Geometry check sheet. Reference: the model listing, model coordinates, mm. Face numbers are marked on the shaded views. A direction names the side the tool comes from. Give positions to 0.01 mm unless a question says otherwise; leave off trailing zeros. Write each loop counter-clockwise with the first axis right and the second up, starting at its lowest first coordinate (ties: lowest second). Pieces come first, ordered by that corner, then holes. Notation, with made-up numbers: M -6.75,27 L -0.75,27 A15 cw -0.75,52 Z; hole C 12.5,5 d9. An arc over 180 degrees is marked long. One line per item, written item: value. Start each with the question number.
1. Cross-section at A-A on z = -3. Record the cut outline in (x, y), then the cut area to 3 significant figures.
2. Tool access check on the marked faces 4 and 5. Record the directions out of +Z, -Z, +X, -X, +Y, -Y that give a thin tool (end or side, any length) a straight path to the whole face; none if there is none.
3. Scan lines: line 1 (Z direction, x = -2, y = -6.75); line 2 (Z direction, x = -2.5, y = -3.75); line 3 (Y direction, x = -0.25, z = -9). Record each from-to range of solid material in increasing order.
4. Release check for a two-part mould opening along Z. For the marked faces 1, 2 and 3 record: pulls with the +Z half, pulls with the -Z half, needs draft (parallel to the pull), parting line crosses it, or undercut.
5. Gauge pin test, flat ends, axial feed: pin 1 (3 mm diameter, centred on y = -1.5, z = -5, fed in from +X); pin 2 (6 mm diameter, centred on x = -4.5, y = 2, fed in from +Z); pin 3 (1 mm diameter, centred on y = 0, z = -4.5, fed in from -X). Record the tip position at first contact, or that the pin passes through.
from build123d import *

# Parameters (mm, degrees)
SKETCH_2_R          = 1.5
CUT_EXTRUDE_1_DEPTH = 24.941073563


with BuildPart() as part:
    # Эскиз1 → Повернуть1 (revolve)
    with BuildSketch(Plane(origin=(0, 0, 0), x_dir=(0, 0, -1), z_dir=(1, 0, 0)), mode=Mode.PRIVATE) as revolve_1_sk:
        with BuildLine():
            Line((-16.75, 0), (16.75, 0))
            Line((16.75, 0), (16.75, 5.5))
            Line((16.75, 5.5), (11.95, 5.5))
            Line((11.95, 5.5), (10.75, 7.65))
            Line((10.75, 7.65), (8.75, 7.65))
            Line((8.75, 7.65), (8.75, 4))
            Line((8.75, 4), (2.45, 4))
            Line((2.45, 4), (2.45, 7.65))
            Line((2.45, 7.65), (1.45, 7.65))
            Line((1.45, 7.65), (1.45, 6.5))
            ThreePointArc((1.45, 6.5), (-6.880526727, 5.027063991), (-14.723327208, 1.855676812))
            ThreePointArc((-14.723327208, 1.855676812), (-15.854421467, 1.056447361), (-16.75, 0))
        make_face()
    revolve(revolve_1_sk.sketch.rotate(Axis((0, 0, -16.75), (0, 0, -1)), 90), axis=Axis((0, 0, -16.75), (0, 0, -1)))

    # Эскиз2 → Вырез-Вытянуть1 (cut, through all)
    with BuildSketch(Plane(origin=(7.65, 0, 0), x_dir=(0, 0, -1), z_dir=(1, 0, 0))):
        with Locations((-11.65, 0)):
            Circle(SKETCH_2_R)
    extrude(amount=-CUT_EXTRUDE_1_DEPTH, mode=Mode.SUBTRACT)


solid = part.part
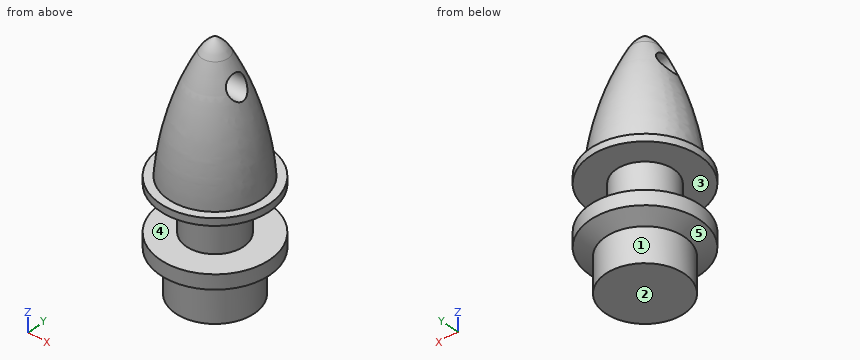
Report:
1. outline: C 0,0 d8
1. area: 50.3 mm^2
2. face 4: none
2. face 5: -Z
3. line 1: z = -11.09 to -8.75, -2.45 to -1.45
3. line 2: z = -16.75 to -8.75, -2.45 to 8.55
3. line 3: y = -7.65 to 7.65
4. face 1: needs draft
4. face 2: pulls with the -Z half
4. face 3: undercut
5. pin 1: stops at x = 4
5. pin 2: stops at z = 14.59
5. pin 3: stops at x = -4
